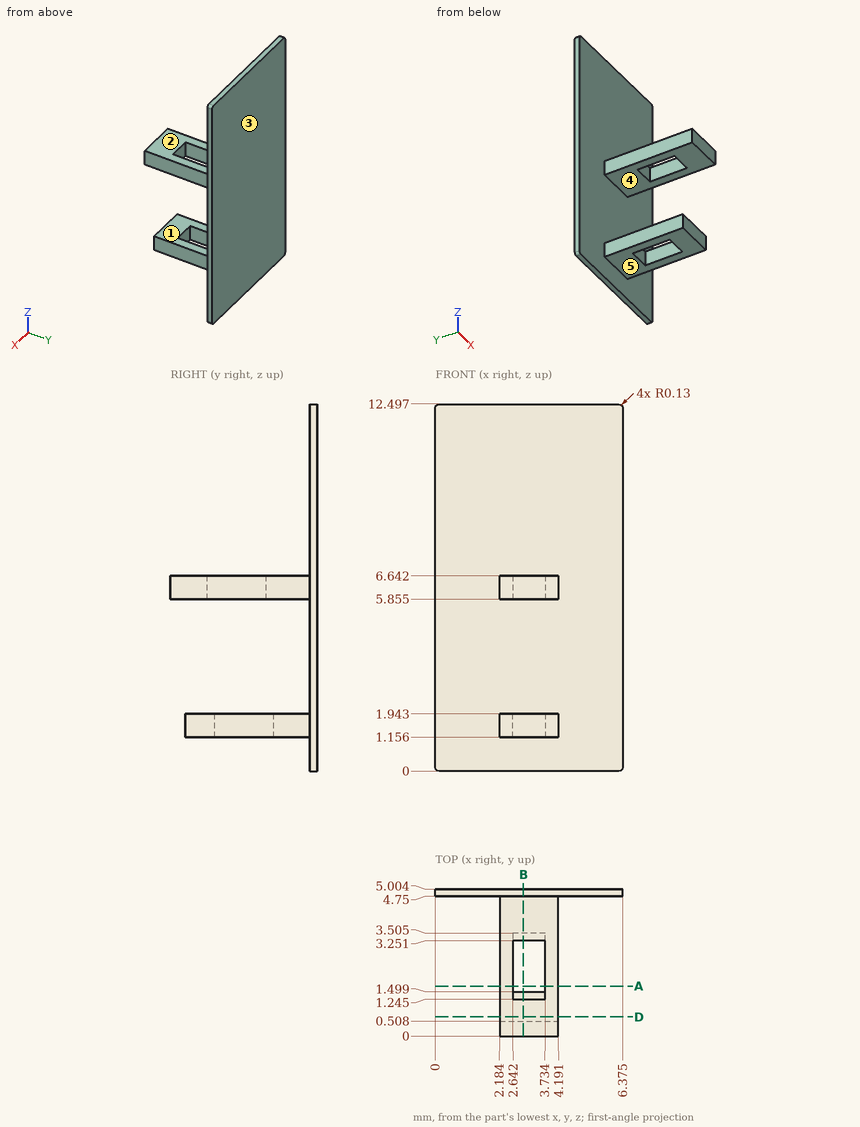
Study the drawing (mm; zero at the part's minimum x, y, z) and answer. A direction names the side the tool comes from. Coordinates: 2 decimals unless noted, no trailing zeros. Order: outer loops, then holes, each group sorted by start corner. A loop starts at its lowest first (then second) coordinate and runs counter-clockwise, first axis right, second up. Notation, with made-up numbers: M -23,35.25 L 12,35.25 A18 cw 12,55.25 Z; hole C 41.25,69.25 d2. An arc over 180 degrees is marked long. Answer as a JSON object with one key per item and string values. Group by question number.
1. Straight lines are drawn through the part: line 1 (Z direction, x = 4, y = 1.9) (1 decimal); line 2 (Y direction, x = 2.5, z = 11.25); line 3 (Z direction, x = 3.5, y = 1.4) (1 decimal). For each, find the intervals that lie inside material, in ascending order.
2. Section B-B on x = 3 is taken. State how many separate pieces and enclosed holes the cut face has.
3. Section A-A on y = 1.7 is taken. Write down the section's boundary in (x, z) (1 decimal).
4. Determine the mould class of the marked faces 1, 2 and 3 for opening direction Z: released by +Z, released by -Z, zero draft, split by the parting line, or undercut.
5. A tool of negligible diameter and unlimited length cuts with its end or side. For the marked faces 4 and 5, from which of +Z, -Z, +X, -X, +Y, -Y can it reach the whole face along a straight path? Write none if from no direction.
6. Section D-D on y = 0.65 is taken. Write down the section's boundary in (x, z) (1 decimal).
7. Flat-ended cylindrical pins translate along their axes: P1, Ø3, axis at x = 2.5, y = 2.5, coming from the +Z side; P2, Ø0.6, axis at y = 2.5, z = 1.5, coming from the +X side; P3, Ø1, axis at x = 3.5, y = 2.5, coming from the -Z side; P4, Ø0.6, axis at x = 3, y = 2.5, coming from the -Z side. Find the tip coordinate at first contact, or state that the pin passes through.
Values follow:
{
 "1": {"line 1": "1.2 to 1.9, 5.9 to 6.6", "line 2": "4.75 to 5", "line 3": "1.2 to 1.9"},
 "2": {"separate pieces": "3", "enclosed holes": "0"},
 "3": {"outline": "M 2.2,1.2 L 2.6,1.2 L 2.6,1.9 L 2.2,1.9 Z; M 2.2,5.9 L 2.6,5.9 L 2.6,6.6 L 2.2,6.6 Z; M 3.7,1.2 L 4.2,1.2 L 4.2,1.9 L 3.7,1.9 Z; M 3.7,5.9 L 4.2,5.9 L 4.2,6.6 L 3.7,6.6 Z"},
 "4": {"face 1": "undercut", "face 2": "released by +Z", "face 3": "zero draft"},
 "5": {"face 4": "+X, -X, -Y", "face 5": "-Z, +X, -X, -Y"},
 "6": {"outline": "M 2.2,1.2 L 4.2,1.2 L 4.2,1.9 L 2.2,1.9 Z; M 2.2,5.9 L 4.2,5.9 L 4.2,6.6 L 2.2,6.6 Z"},
 "7": {"P1": "z = 6.64", "P2": "x = 4.19", "P3": "z = 1.16", "P4": "through"}
}
